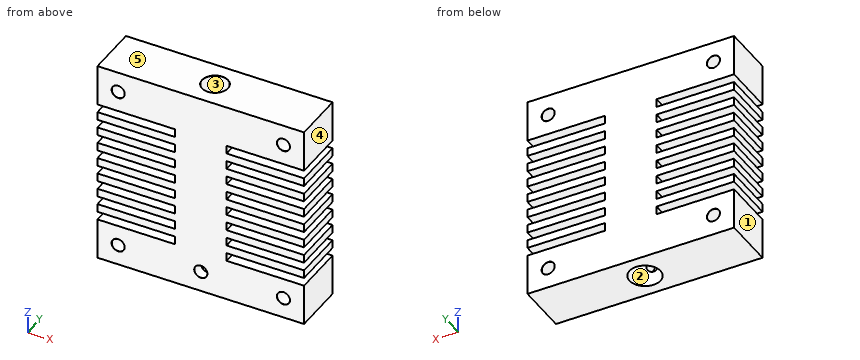
from build123d import *

# Parameters (mm, degrees)
ESQUISSE1_W                                         = 40
ESQUISSE1_H                                         = 40
BOSS_EXTRU_1_DEPTH                                  = 10
DIAM_TRE_DU_PER_AGE_4_0_4_1_D                       = 4
TROU_POUR_TARAUDAGE_POUR_TROU_TARAUD_M6_D           = 5
TROU_POUR_TARAUDAGE_POUR_TROU_TARAUD_M6_DEPTH       = 8
TROU_POUR_TARAUDAGE_POUR_TROU_TARAUD_M6_CSINK_D     = 5.05
TROU_POUR_TARAUDAGE_POUR_TROU_TARAUD_M6_CSINK_ANGLE = 90
TROU_POUR_TARAUDAGE_POUR_TROU_TARAUD_M6_TIP         = 1.502151548
DIAM_TRE_DU_PER_AGE_6_0_6_1_D                       = 6
DIAM_TRE_DU_PER_AGE_6_0_6_1_DEPTH                   = 20
DIAM_TRE_DU_PER_AGE_6_0_6_1_TIP                     = 1.802581857
TROU_POUR_TARAUDAGE_POUR_TROU_TARAUD_2_COUNT        = 2
TROU_POUR_TARAUDAGE_POUR_TROU_TARAUD_2_PITCH        = 32
TROU_POUR_TARAUDAGE_POUR_TROU_TARAUD_3_COUNT        = 2
TROU_POUR_TARAUDAGE_POUR_TROU_TARAUD_3_PITCH        = 45.254833996
TROU_POUR_TARAUDAGE_POUR_TROU_TARAUD_4_COUNT        = 2
TROU_POUR_TARAUDAGE_POUR_TROU_TARAUD_4_PITCH        = 32
TROU_POUR_TARAUDAGE_POUR_TROU_TARAUD_5_D            = 2.5
TROU_POUR_TARAUDAGE_POUR_TROU_TARAUD_5_DEPTH        = 5
TROU_POUR_TARAUDAGE_POUR_TROU_TARAUD_5_CSINK_D      = 2.55
TROU_POUR_TARAUDAGE_POUR_TROU_TARAUD_5_CSINK_ANGLE  = 90
TROU_POUR_TARAUDAGE_POUR_TROU_TARAUD_5_TIP          = 0.751075774
ESQUISSE21_W                                        = 15
ESQUISSE21_H                                        = 1.6
ENL_V_MAT_EXTRU_1_DEPTH                             = 58.445626535
R_P_TITION_LIN_AIRE1_COUNT                          = 8
R_P_TITION_LIN_AIRE1_PITCH                          = 3.2


with BuildPart() as part:
    # Esquisse1 → Boss.-Extru.1 (new body)
    with BuildSketch(Plane(origin=(0, 0, 0), x_dir=(1, 0, 0), z_dir=(0, 1, 0))):
        with Locations((20, 20)):
            Rectangle(ESQUISSE1_W, ESQUISSE1_H)
    extrude(amount=BOSS_EXTRU_1_DEPTH)

    # Diamètre du perçage Ø4.0 (4)1 (through all)
    with Locations(Plane.XY):
        with Locations((20, 5)):
            Hole(DIAM_TRE_DU_PER_AGE_4_0_4_1_D / 2)

    # Trou pour taraudage pour trou taraudé M61
    with Locations(Plane.XY):
        with Locations((20, 5)):
            CounterSinkHole(TROU_POUR_TARAUDAGE_POUR_TROU_TARAUD_M6_D / 2, TROU_POUR_TARAUDAGE_POUR_TROU_TARAUD_M6_CSINK_D / 2, depth=TROU_POUR_TARAUDAGE_POUR_TROU_TARAUD_M6_DEPTH, counter_sink_angle=TROU_POUR_TARAUDAGE_POUR_TROU_TARAUD_M6_CSINK_ANGLE)
            with Locations((0, 0, -(TROU_POUR_TARAUDAGE_POUR_TROU_TARAUD_M6_DEPTH + TROU_POUR_TARAUDAGE_POUR_TROU_TARAUD_M6_TIP / 2))):  # 118° drill point
                Cone(0, TROU_POUR_TARAUDAGE_POUR_TROU_TARAUD_M6_D / 2, TROU_POUR_TARAUDAGE_POUR_TROU_TARAUD_M6_TIP, mode=Mode.SUBTRACT)

    # Diamètre du perçage Ø6.0 (6)1
    with Locations(Plane(origin=(0, 0, -40), x_dir=(-1, 0, 0), z_dir=(0, 0, -1))):
        with Locations((-20, 5)):
            Hole(DIAM_TRE_DU_PER_AGE_6_0_6_1_D / 2, depth=DIAM_TRE_DU_PER_AGE_6_0_6_1_DEPTH)
            with Locations((0, 0, -(DIAM_TRE_DU_PER_AGE_6_0_6_1_DEPTH + DIAM_TRE_DU_PER_AGE_6_0_6_1_TIP / 2))):  # 118° drill point
                Cone(0, DIAM_TRE_DU_PER_AGE_6_0_6_1_D / 2, DIAM_TRE_DU_PER_AGE_6_0_6_1_TIP, mode=Mode.SUBTRACT)

    # Esquisse17 → Trou pour taraudage pour trou taraud_ M3 (revolve, cut)
    with BuildSketch(Plane(origin=(4, 0, -4), x_dir=(0, 0, -1), z_dir=(1, 0, 0))):
        Polygon((0, 0), (0, 10), (1.275, 10), (1.25, 9.975), (1.25, 0.025), (1.275, 0), align=None)
    trou_pour_taraudage_pour_trou_taraud_m3 = revolve(axis=Axis((4, -6.35, -4), (0, 1, 0)), mode=Mode.SUBTRACT)

    # Trou pour taraudage pour trou taraud 2: Trou pour taraudage pour trou taraud_ M3 ×2
    with Locations(*[(i * TROU_POUR_TARAUDAGE_POUR_TROU_TARAUD_2_PITCH, 0, 0) for i in range(1, TROU_POUR_TARAUDAGE_POUR_TROU_TARAUD_2_COUNT)]):
        add(trou_pour_taraudage_pour_trou_taraud_m3, mode=Mode.SUBTRACT)

    # Trou pour taraudage pour trou taraud 3: Trou pour taraudage pour trou taraud_ M3 ×2
    with Locations(*[Vector(0.7071067811865475, 0, -0.7071067811865476) * (i * TROU_POUR_TARAUDAGE_POUR_TROU_TARAUD_3_PITCH) for i in range(1, TROU_POUR_TARAUDAGE_POUR_TROU_TARAUD_3_COUNT)]):
        add(trou_pour_taraudage_pour_trou_taraud_m3, mode=Mode.SUBTRACT)

    # Trou pour taraudage pour trou taraud 4: Trou pour taraudage pour trou taraud_ M3 ×2
    with Locations(*[(0, 0, -i * TROU_POUR_TARAUDAGE_POUR_TROU_TARAUD_4_PITCH) for i in range(1, TROU_POUR_TARAUDAGE_POUR_TROU_TARAUD_4_COUNT)]):
        add(trou_pour_taraudage_pour_trou_taraud_m3, mode=Mode.SUBTRACT)

    # Trou pour taraudage pour trou taraud 5
    with Locations(Plane(origin=(0, 0, 0), x_dir=(-1, 0, 0), z_dir=(0, -1, 0))):
        with Locations((-20, 36)):
            CounterSinkHole(TROU_POUR_TARAUDAGE_POUR_TROU_TARAUD_5_D / 2, TROU_POUR_TARAUDAGE_POUR_TROU_TARAUD_5_CSINK_D / 2, depth=TROU_POUR_TARAUDAGE_POUR_TROU_TARAUD_5_DEPTH, counter_sink_angle=TROU_POUR_TARAUDAGE_POUR_TROU_TARAUD_5_CSINK_ANGLE)
            with Locations((0, 0, -(TROU_POUR_TARAUDAGE_POUR_TROU_TARAUD_5_DEPTH + TROU_POUR_TARAUDAGE_POUR_TROU_TARAUD_5_TIP / 2))):  # 118° drill point
                Cone(0, TROU_POUR_TARAUDAGE_POUR_TROU_TARAUD_5_D / 2, TROU_POUR_TARAUDAGE_POUR_TROU_TARAUD_5_TIP, mode=Mode.SUBTRACT)

    # Esquisse21 → Enlèv. mat.-Extru.1 (cut, through all)
    with BuildSketch(Plane.XZ):
        with Locations((7.5, -8.8)):
            Rectangle(ESQUISSE21_W, ESQUISSE21_H)
        with Locations((32.5, -8.8)):
            Rectangle(ESQUISSE21_W, ESQUISSE21_H)
    enl_v_mat_extru_1 = extrude(amount=-ENL_V_MAT_EXTRU_1_DEPTH, mode=Mode.SUBTRACT)

    # Répétition linéaire1: Enlèv. mat.-Extru.1 ×8
    with Locations(*[(0, 0, -i * R_P_TITION_LIN_AIRE1_PITCH) for i in range(1, R_P_TITION_LIN_AIRE1_COUNT)]):
        add(enl_v_mat_extru_1, mode=Mode.SUBTRACT)


solid = part.part
Build history of the part. All positions in model axes, mm. Face numbers are marked on the shaded views. A direction names the side the tool comes from. Round coordinates to 2 decimals unless told otherwise and drop trailing zeros. Order: outer loops, then holes, each group sorted by start corner. A loop starts at its lowest first (then second) coordinate and runs counter-clockwise, first axis right, second up. Notation, with made-up numbers: M 49.5,-15.75 L 95.5,-15.75 A20 ccw 95.5,3.25 Z; hole C 61,-25.75 d11. An arc over 180 degrees is marked long. Use CSV: the item, a comma, the result in double quotes. Start each with the question number.
(1) Tool access for the marked faces 1 and 2: list every direction of +Z, -Z, +X, -X, +Y, -Y with a clear straight run to the whole face (end or side of a thin tool).
(2) Drill centre lines: probe 1 along X at (y, z) = (5, -36); probe 2 along X at (y, z) = (7.75, -4); probe 3 along X at (y, z) = (5, -11). Where is each one in solid material? Low to high.
(3) Cut at B-B on x = 20. List the corners of the cut face in (y, z) (3 decimals).
(4) Flat gauge pins, fed straight in: P1, Ø0.8, axis at y = 4, z = -31, coming from the +X side; P2, Ø1.3, axis at y = 5, z = -12, coming from the -X side. Where does each tip first touch, or does it go through?
(5) Cut at C-C on y = 5. State how many separate pieces and enclosed holes the cut face has, then the cut area to 3 significant figures.
(6) Cut at D-D on z = -36. List the corners of the cut face in (x, y) (3 decimals), then the cut area to 4 significant figures.
(7) Cut at A-A on z = -4. List the corners of the cut face in (x, y) (3 decimals), then the cut area to 3 significant figures.
(8) Mould opens along X. For the marked faces 3, 4 and 5 say: +X half, -X half, draft (parallel to the pull), parting line (faces both ways), or undercut.
Findings:
1,face 1,"+Z, -Z, -X, +Y, -Y"
1,face 2,"-Z"
2,probe 1,"x = 0 to 2.75, 5.25 to 17, 23 to 34.75, 37.25 to 40"
2,probe 2,"x = 0 to 2.75, 5.25 to 34.75, 37.25 to 40"
2,probe 3,"x = 0 to 18, 22 to 40"
3,outline,"M 0,-40 L 2,-40 L 2,-37.25 L 0.025,-37.25 L 0,-37.275 Z; M 0,-34.725 L 0.025,-34.75 L 2,-34.75 L 2,-20 L 3,-19.399 L 3,-8.3 L 2.5,-8 L 2.5,-0.025 L 2.475,0 L 0,0 Z; M 7,-19.399 L 8,-20 L 8,-40 L 10,-40 L 10,0 L 7.525,0 L 7.5,-0.025 L 7.5,-8 L 7,-8.3 Z"
4,P1,"stops at x = 25"
4,P2,"stops at x = 15"
5,separate pieces,"2"
5,enclosed holes,"4"
5,area,"988 mm^2"
6,outline,"M 0,0 L 2.725,0 L 2.75,0.025 L 2.75,9.975 L 2.725,10 L 0,10 Z; M 5.25,0.025 L 5.275,0 L 18.725,0 L 18.75,0.025 L 18.75,2.273 A3 cw long 21.25,2.273 L 21.25,0.025 L 21.275,0 L 34.725,0 L 34.75,0.025 L 34.75,9.975 L 34.725,10 L 5.275,10 L 5.25,9.975 Z; M 37.25,0.025 L 37.275,0 L 40,0 L 40,10 L 37.275,10 L 37.25,9.975 Z"
6,area,"316.5 mm^2"
7,outline,"M 0,0 L 2.725,0 L 2.75,0.025 L 2.75,9.975 L 2.725,10 L 0,10 Z; M 5.25,0.025 L 5.275,0 L 34.725,0 L 34.75,0.025 L 34.75,9.975 L 34.725,10 L 5.275,10 L 5.25,9.975 Z; M 37.25,0.025 L 37.275,0 L 40,0 L 40,10 L 37.275,10 L 37.25,9.975 Z; hole C 20,5 d5"
7,area,"330 mm^2"
8,face 3,"undercut"
8,face 4,"+X half"
8,face 5,"draft"
